Work out the finished part from the listing and answer in its coordinate system (mm). A direction names the side the tool comes from. Round coordinates to 2 decimals unless told otherwise and drop trailing zeros. Order: outer loops, then holes, each group sorted by start corner. A loop starts at its lowest first (then second) coordinate and runs counter-clockwise, first axis right, second up. Notation, with made-up numbers: (-13.75, 25.5) - (22.25, 25.5) arc R20 ccw to (22.25, 57.5) - close; hole circle Ø4 at (-34, 77.25). An arc over 180 degrees is marked (long way). Put each result on its own line as item: value.
```python
from build123d import *

# Parameters (mm, degrees)
BOSS_EXTRUDE1_DEPTH = 10
BOSS_EXTRUDE2_DEPTH = 30
CUT_EXTRUDE1_REACH  = 37
CUT_EXTRUDE2_REACH  = 12
SKETCH3_R           = 4
FILLET1_R           = 10
FILLET2_R           = 8
CUT_EXTRUDE3_REACH  = 12
SKETCH4_R           = 4


with BuildPart() as part:
    # Sketch1 → Boss-Extrude1 (new body)
    with BuildSketch(Plane(origin=(0, 0, 0), x_dir=(1, 0, 0), z_dir=(0, 1, 0))):
        Polygon((40, 0), (40, 30), (20, 30), (20, 5), (0, 5), (0, 0), align=None)
    extrude(amount=BOSS_EXTRUDE1_DEPTH)

    # Sketch1_3 → Boss-Extrude2 (add)
    with BuildSketch(Plane(origin=(0, 0, 0), x_dir=(1, 0, 0), z_dir=(0, 1, 0))):
        Polygon((20, 30), (40, 30), (40, 40), (0, 40), (0, 5), (20, 5), align=None)
    extrude(amount=BOSS_EXTRUDE2_DEPTH)

    # Sketch2 → Cut-Extrude1 (cut, up to next)
    with BuildSketch(Plane.XY.offset(-5), mode=Mode.PRIVATE) as cut_extrude1_sk1:
        with BuildLine():
            Line((15, 30), (0, 30))
            Line((0, 30), (0, 15))
            ThreePointArc((0, 15), (10.606601718, 19.393398282), (15, 30))
        make_face()
    cut_extrude1_tool1 = extrude(cut_extrude1_sk1.sketch, amount=-CUT_EXTRUDE1_REACH, mode=Mode.PRIVATE) & part.part
    add(cut_extrude1_tool1.solids().sort_by_distance((6.366198, 23.633802, -5))[0], mode=Mode.SUBTRACT)

    # Sketch3 → Cut-Extrude2 (cut, up to next)
    with BuildSketch(Plane(origin=(0, 10, 0), x_dir=(1, 0, 0), z_dir=(0, 1, 0)), mode=Mode.PRIVATE) as cut_extrude2_sk1:
        with Locations((30, 10)):
            Circle(SKETCH3_R)
    cut_extrude2_tool1 = extrude(cut_extrude2_sk1.sketch, amount=-CUT_EXTRUDE2_REACH, mode=Mode.PRIVATE) & part.part
    add(cut_extrude2_tool1.solids().sort_by_distance((30, 10, -10))[0], mode=Mode.SUBTRACT)

    # Fillet1
    fillet1_edges = [part.edges().sort_by_distance(p)[0] for p in [
        (40, 5, 0),
    ]]
    fillet(fillet1_edges, radius=FILLET1_R)

    # Fillet2
    fillet2_edges = [part.edges().sort_by_distance(p)[0] for p in [
        (40, 30, -35),
    ]]
    fillet(fillet2_edges, radius=FILLET2_R)

    # Sketch4 → Cut-Extrude3 (cut, up to next)
    with BuildSketch(Plane.XY.offset(-30), mode=Mode.PRIVATE) as cut_extrude3_sk1:
        with Locations((32, 22)):
            Circle(SKETCH4_R)
    cut_extrude3_tool1 = extrude(cut_extrude3_sk1.sketch, amount=-CUT_EXTRUDE3_REACH, mode=Mode.PRIVATE) & part.part
    add(cut_extrude3_tool1.solids().sort_by_distance((32, 22, -30))[0], mode=Mode.SUBTRACT)

    # Mirror1: part across plane


with BuildPart() as part_1:
    add(part.part)
    add(part.part.mirror(Plane(origin=(0, 10, 0), x_dir=(0, 0, 1), z_dir=(-1, 0, 0))))


solid = part_1.part
```
1) Given pin 1 Ø9 at (x, z) = (30, -10) entering from +Y; pin 2 Ø10 at (x, y) = (19, 24) entering from +Z; pin 3 Ø5 at (y, z) = (16.5, -7.5) entering from +X, each flat-ended and moving along its own axis, determine where each tip first touches the part or whether it passes through.
Findings below:
pin 1: stops at y = 10
pin 2: stops at z = -5
pin 3: stops at x = 20
2) Straight lines are drawn through the part: L1, parallel to Z at x = 30, y = 2.75; L2, parallel to Y at x = 32, z = -32.5; L3, parallel to Y at x = -30, z = -15. For each, find the intervals that lie inside material, in ascending order. Write a range as from..to.
Findings below:
L1: z = -40..-14, -6..0
L2: y = 0..18, 26..30
L3: y = 0..10
3) A cutting plane is placed at B-B on y = 8.75. Write down the section's boundary in (x, z).
Findings below:
outline: (-40, -40) - (40, -40) - (40, -10) arc R10 ccw to (30, 0) - (-30, 0) arc R10 ccw to (-40, -10) - close; hole circle Ø8 at (-30, -10); hole circle Ø8 at (30, -10)
4) For a pull along Z with two mould halves and no side action, classify faces 4 (the flat face through (1, 10, -2)), 5 (the cylindrical face through (26, 5, -10)), 6 (the flat face through (0, 13, -5)) as pulls with the +Z half, pulls with the -Z half, needs draft (parallel to the pull), parting line crosses it, or undercut.
Findings below:
face 4: needs draft
face 5: undercut
face 6: pulls with the +Z half
5) A cutting plane is placed at D-D on z = -8. Write down the section's boundary in (x, y), then the cut area to 3 significant figures.
Findings below:
outline: (-39.8, 0) - (-33.46, 0) - (-33.46, 10) - (-39.8, 10) - close; (-26.54, 0) - (26.54, 0) - (26.54, 10) - (20, 10) - (20, 30) - (15, 30) arc R15 cw to (-15, 30) - (-20, 30) - (-20, 10) - (-26.54, 10) - close; (33.46, 0) - (39.8, 0) - (39.8, 10) - (33.46, 10) - close
area: 1,100 mm2
6) For faces 1 (the flat face through (-28, 20, -30)), 2 (the cylindrical face through (31.479, 25.966, -34.93)), 3 (the flat face through (28, 20, -30)), determine the directions among +Z, -Z, +X, -X, +Y, -Y from which every point of the face is accessible in a straight line to the end or side of a thin tool.
Findings below:
face 1: +Z, -X, +Y
face 2: +Z, -Z
face 3: +Z, +X, +Y
7) A cutting plane is placed at A-A on z = -32. Write down the section's boundary in (x, y), then the cut area to 3 significant figures.
Findings below:
outline: (-40, 0) - (40, 0) - (40, 22) arc R8 ccw to (32, 30) - (15, 30) arc R15 cw to (-15, 30) - (-32, 30) arc R8 ccw to (-40, 22) - close; hole circle Ø8 at (-32, 22); hole circle Ø8 at (32, 22)
area: 1,920 mm2
8) A cutting plane is placed at C-C on y = 28. Write down the section's boundary in (x, z).
Findings below:
outline: (-37.29, -40) - (-14.87, -40) - (-14.87, -5) - (-20, -5) - (-20, -30) - (-37.29, -30) - close; (14.87, -40) - (37.29, -40) - (37.29, -30) - (20, -30) - (20, -5) - (14.87, -5) - close
